Geometry check sheet. Reference: the model listing, model coordinates, mm. A direction names the side the tool comes from. Coordinates: 2 decimals unless noted, no trailing zeros. Loops run counter-clockwise (first coordinate to the right, second up) from the corner with the lowest first, then second, coordinate; pieces in that order, holes last. Notation, with made-up numbers: (31, 39) - (40, 39) arc R19 ccw to (40, 64) - close; hole circle Ø9 at (-0.5, 13). An arc over 180 degrees is marked (long way). One line per item, written item: value.
from build123d import *

# Parameters (mm, degrees)
SKETCH2_R          = 2.571129816
CUT_EXTRUDE2_DEPTH = 25.4


with BuildPart() as part:
    # Sketch1 → Revolve-Thin3 (revolve)
    with BuildSketch(Plane.XY):
        Polygon((0.497679461, 0), (8.560086725, 0), (8.560086725, 10.16), (4.379579254, 10.16), (4.379579254, 25.527), (8.560086725, 25.527), (8.560086725, 35.687), (-8.560086725, 35.687), (-8.560086725, 25.527), (-4.379579254, 25.527), (-4.379579254, 10.16), (-8.560086725, 10.16), (-8.560086725, 0), (-0.497679461, 0), (-0.497679461, 0.254), (-8.306086725, 0.254), (-8.306086725, 9.906), (-4.125579254, 9.906), (-4.125579254, 25.781), (-8.306086725, 25.781), (-8.306086725, 35.433), (8.306086725, 35.433), (8.306086725, 25.781), (4.125579254, 25.781), (4.125579254, 9.906), (8.306086725, 9.906), (8.306086725, 0.254), (0.497679461, 0.254), align=None)
    revolve(axis=Axis((-8.560086725, 0, 0), (1, 0, 0)))

    # Sketch2 → Cut-Extrude2 (cut)
    with BuildSketch(Plane.ZY.offset(8.560086725)):
        Circle(SKETCH2_R)
    extrude(amount=-CUT_EXTRUDE2_DEPTH, mode=Mode.SUBTRACT)


solid = part.part
(1) Cross-section at B-B on z = -23.5. Record the cut outline in (x, y), and give its area (3 significant figures).
Reply:
outline: (-8.56, -26.86) - (8.56, -26.86) - (8.56, -9.97) - (4.38, -9.97) - (4.38, 9.97) - (8.56, 9.97) - (8.56, 26.86) - (-8.56, 26.86) - (-8.56, 9.97) - (-4.38, 9.97) - (-4.38, -9.97) - (-8.56, -9.97) - close; hole (-8.31, -26.52) - (8.31, -26.52) - (8.31, -10.6) - (4.13, -10.6) - (4.13, 10.6) - (8.31, 10.6) - (8.31, 26.52) - (-8.31, 26.52) - (-8.31, 10.6) - (-4.13, 10.6) - (-4.13, -10.6) - (-8.31, -10.6) - close
area: 49.1 mm2
(2) Access from +Z, -Z, +X, -X, +Y, -Y to the whole of each face (thin tool, end or side, straight path). Record for faces 4 (the face through (-8.56, -8.4, 24.3)), 5 (the face through (-4.38, 11, 0)), 6 (the face through (0.12, -7.68, -34.59)), 7 (the face through (6.499, 24.348, 7.668)).
Reply:
face 4: +Z, -Z, -X, +Y, -Y
face 5: -X
face 6: none
face 7: +X
(3) Material ranges on probe 1 along Z at (x, y) = (6.4, 0); probe 2 along X at (y, z) = (-29.5, 6.5); probe 3 along Z at (x, y) = (5, -10.5), recorded low to high. Write a range as from..to.
Reply:
probe 1: -35.69..-35.43, -25.78..-25.53, -10.16..-9.91, 9.91..10.16, 25.53..25.78, 35.43..35.69
probe 2: -8.56..-8.31, 8.31..8.56
probe 3: -34.11..-33.84, -23.55..-23.27, 23.27..23.55, 33.84..34.11
(4) Cross-section at A-A on y = -19. Record the cut outline in (x, z).
Reply:
outline: (-8.56, -30.21) - (8.56, -30.21) - (8.56, -17.05) - (4.38, -17.05) - (4.38, 17.05) - (8.56, 17.05) - (8.56, 30.21) - (-8.56, 30.21) - (-8.56, 17.05) - (-4.38, 17.05) - (-4.38, -17.05) - (-8.56, -17.05) - close; hole (-8.31, -29.91) - (8.31, -29.91) - (8.31, -17.43) - (4.13, -17.43) - (4.13, 17.43) - (8.31, 17.43) - (8.31, 29.91) - (-8.31, 29.91) - (-8.31, 17.43) - (-4.13, 17.43) - (-4.13, -17.43) - (-8.31, -17.43) - close
(5) Cross-section at D-D on z = 27.5. Record the cut outline in (x, y), and give its area (3 significant figures).
Reply:
outline: (-8.56, -22.74) - (8.56, -22.74) - (8.56, 22.74) - (-8.56, 22.74) - close; hole (-8.31, -22.34) - (8.31, -22.34) - (8.31, 22.34) - (-8.31, 22.34) - close
area: 36.4 mm2
(6) Go/stop test with flat-tipped pins: pin 1 Ø3 at (y, z) = (2, 21.5) entering from +X; pin 2 Ø5 at (x, z) = (-0.5, -11.5) entering from -Y; pin 3 Ø10 at (x, z) = (5.5, 9) entering from +Y; pin 4 Ø4.5 at (y, z) = (0, 0) entering from -X. Record where each tip stops, or that it passes through.
Reply:
pin 1: x = 4.38
pin 2: y = -34.53
pin 3: y = 35.46
pin 4: through
(7) Cross-section at C-C on x = -1.5. Record the cut outline in (y, z).
Reply:
outline: circle Ø71.37 at (0, 0); hole circle Ø70.87 at (0, 0)
(8) Release check for a two-part mould opening along Y. For faces 1 (the face through (8.56, 8.4, 24.3)), 2 (the face through (-0.12, 19.19, 30.09)), 3 (the face through (-6.19, -1.29, 9.82)) record: pulls with the +Y half, pulls with the -Y half, needs draft (parallel to the pull), parting line crosses it, or undercut.
Reply:
face 1: needs draft
face 2: parting line crosses it
face 3: undercut
